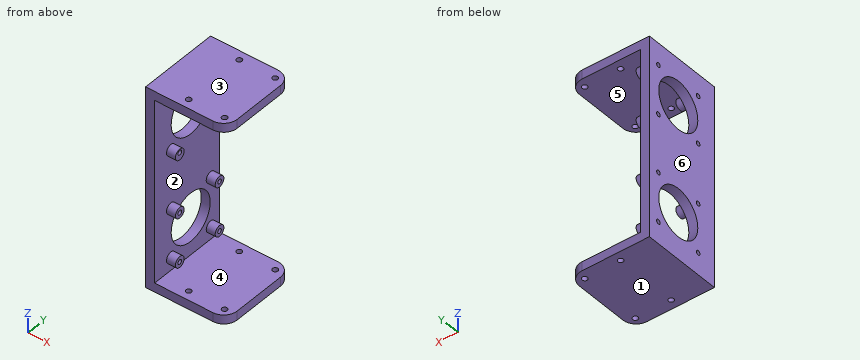
Autodesk Inventor part; units mm, degrees
ref_plane "Work Plane2" through (0, 0, 56) normal (0, 0, -1) x (-1, 0, 0)
ref_plane "YZ Plane" through (0, 0, 0) normal (1, 0, 0) x (0, 1, 0)
ref_plane "XZ Plane" through (0, 0, 0) normal (0, 1, 0) x (-1, 0, 0)
sketch "Sketch1" plane through (0, 0, 0) normal (0, 0, 1) x (1, 0, 0)
  line L0 (0, 0) -> (20, 0)
  line L1 (20, 0) -> (20, 35)
  line L2 (20, 35) -> (0, 35)
  line L3 (0, 35) -> (0, 0)
  circle A0 centre (0, 35) radius 1.5
  circle A1 centre (20, 35) radius 1.5
  circle A2 centre (0, 0) radius 1.5
  circle A3 centre (20, 0) radius 1.5
  line L4 (0, 35) -> (20, 0)
  line L5 (-15, -5) -> (20, -5)
  line L6 (20, -5) -> (20, 40)
  line L7 (20, 40) -> (-15, 40)
  line L8 (-15, 40) -> (-15, -5)
  line L9 (20, 40) -> (25, 40)
  line L10 (25, 40) -> (25, -5)
  line L11 (25, -5) -> (20, -5)
  line L12 (20, -5) -> (20, 40)
  point P0 (10, 17.5)
  point P1 (20, 36.5)
  point P2 (20, 33.5)
  point P3 (20, 1.5)
  point P4 (20, -1.5)
  dimension "d0" = 35
  dimension "d1" = 20
  dimension "d2" = 3
  dimension "d3" = 3
  dimension "d4" = 3
  dimension "d5" = 3
  dimension "d6" = 5
  dimension "d7" = 15
  dimension "d45" = 5
  dimension "d46" = 45
  dimension "d47" = 10
extrude "Extrusion1" add sketch "Sketch1" along normal blind 5 contours A2 L3 A0 L4 A3 L0 | L0 A3 L6 L5 L8 L7 A1 L2 A0 L3 A2 | L4 A0 L2 A1 L1 A3 | A3 L1 A1 L6 L9 L10 L11
sketch "Sketch2" plane through (0, 0, 5) normal (0, 0, 1) x (1, 0, 0)
  line L0 (30, 40) -> (-15, 40)
  line L1 (-15, 40) -> (-20, 40)
  line L2 (-20, 40) -> (-20, -5)
  line L3 (-20, -5) -> (-15, -5)
  line L4 (-15, -5) -> (-15, 40)
  point P0 (0, 0)
  dimension "d10" = 5
extrude "Extrusion2" add sketch "Sketch2" along normal blind 107 and the other way blind 5
ref_plane "Work Plane2" through (0, 0, 56) normal (0, 0, -1) x (-1, 0, 0)
mirror "Mirror2" about plane through (0, 0, 56) normal (0, 0, -1) of "Extrusion1"
sketch "Sketch3" plane through (-15, -5, 5) normal (1, 0, 0) x (0, 0, -1)
  line L0 (-102, 45) -> (-102, 0)
  line L1 (-102, 25) -> (0, 25)
  line L2 (0, 45) -> (0, 0)
  circle A0 centre (-81, 25) radius 13.5
  circle A1 centre (-21, 25) radius 13.5
  line L3 (-94.75, 38.75) -> (-67.25, 38.75)
  line L4 (-67.25, 38.75) -> (-67.25, 11.25)
  line L5 (-67.25, 11.25) -> (-94.75, 11.25)
  line L6 (-94.75, 11.25) -> (-94.75, 38.75)
  line L7 (-94.75, 38.75) -> (-67.25, 11.25) construction
  line L8 (-67.25, 38.75) -> (-94.75, 11.25) construction
  line L9 (0, 45) -> (-102, 45)
  line L10 (-7.25, 11.25) -> (-34.75, 11.25)
  line L11 (-34.75, 11.25) -> (-34.75, 38.75)
  line L12 (-34.75, 38.75) -> (-7.25, 38.75)
  line L13 (-7.25, 38.75) -> (-7.25, 11.25)
  line L14 (-7.25, 11.25) -> (-34.75, 38.75) construction
  line L15 (-34.75, 11.25) -> (-7.25, 38.75) construction
  circle A2 centre (-94.75, 38.75) radius 3
  circle A3 centre (-67.25, 38.75) radius 3
  circle A4 centre (-67.25, 11.25) radius 3
  circle A5 centre (-94.75, 11.25) radius 3
  circle A6 centre (-34.75, 38.75) radius 3
  circle A7 centre (-7.25, 38.75) radius 3
  circle A8 centre (-7.25, 11.25) radius 3
  circle A9 centre (-34.75, 11.25) radius 3
  circle A10 centre (-94.75, 38.75) radius 1.25
  circle A11 centre (-67.25, 38.75) radius 1.25
  circle A12 centre (-68.25, 11.25) radius 1.25
  circle A13 centre (-94.75, 11.25) radius 1.25
  circle A14 centre (-34.75, 38.75) radius 1.25
  circle A15 centre (-7.25, 38.75) radius 1.25
  circle A16 centre (-34.75, 11.25) radius 1.25
  circle A17 centre (-7.25, 11.25) radius 1.25
  point P0 (5, 5)
  dimension "d16" = 27
  dimension "d17" = 27
  dimension "d18" = 27.5
  dimension "d19" = 27.5
  dimension "d20" = 20
  dimension "d21" = 21
  dimension "d22" = 21
  dimension "d23" = 27.5
  dimension "d24" = 27.5
  dimension "d25" = 6
  dimension "d26" = 6
  dimension "d27" = 6
  dimension "d28" = 6
  dimension "d29" = 6
  dimension "d30" = 6
  dimension "d31" = 6
  dimension "d32" = 6
  dimension "d33" = 2.5
  dimension "d34" = 2.5
  dimension "d35" = 2.5
  dimension "d36" = 2.5
  dimension "d37" = 2.5
  dimension "d38" = 2.5
  dimension "d39" = 2.5
  dimension "d40" = 2.5
extrude "Extrusion3" cut sketch "Sketch3" against normal blind 6 contours A0 L1 | L1 A0 | A13 L5 L6 | L6 L5 A13 | A10 L3 L6 | L6 L3 A10 | A1 L1 | L1 A1 | A15 L12 L13 | L13 L12 A15 | A17 L10 L13 | L13 L10 A17 | A12 L4 L5 | L5 L4 A12 | A11 L4 L3 | L3 L4 A11 | A14 L11 L12 | L12 L11 A14 | A16 L11 L10 | L10 L11 A16
extrude "Extrusion4" add sketch "Sketch3" along normal blind 5 contours A5 L5 A13 L6 | L6 A13 L5 A5 | A2 L3 A10 L6 | L6 A10 L3 A2 | A7 L12 A15 L13 | L13 A15 L12 A7 | A8 L10 A17 L13 | L13 A17 L10 A8 | A4 L4 A12 L5 | L5 A12 L4 A4 | A3 L4 A11 L3 | L3 A11 L4 A3 | A6 L11 A14 L12 | L12 A14 L11 A6 | A9 L11 A16 L10 | L10 A16 L11 A9
fillet "Fillet2" radius 7.5 4 edges at (25, 40, 2.5) (25, -5, 2.5) (25, -5, 109.5) (25, 40, 109.5)
equation "\"d41\" = d30"
properties part number "StereoVisionHolder_3"
Verification items for the finished model (mm, model axes). Face numbers are marked on the shaded views. A direction names the side the tool comes from. Give positions to 0.01 mm unless a question says otherwise; leave off trailing zeros. Order: outer loops, then holes, each group sorted by start corner. A loop starts at its lowest first (then second) coordinate and runs counter-clockwise, first axis right, second up. Notation, with made-up numbers: (15, 13.5) - (58, 13.5) arc R15 cw to (58, 38.5) - close; hole circle Ø11 at (48, -30.75). An arc over 180 degrees is marked (long way). Answer as CSV lines item,"result". Start each with the question number.
Item 1: Gauge pin test, flat ends, axial feed: pin 1 (8 mm diameter, centred on x = -2.5, y = 11, fed in from -Z); pin 2 (2.5 mm diameter, centred on x = 20, y = 0, fed in from -Z); pin 3 (1.8 mm diameter, centred on y = 5, z = 39.5, fed in from +X); pin 4 (1.5 mm diameter, centred on y = 23, z = 57, fed in from +X). Record the tip position at first contact, or that the pin passes through.
Item 2: Section check C-C, the plane z = 26. Record the boundary of the cut face in (x, y), plus the area to 3 significant figures.
Item 3: Section check D-D, the plane y = 0. Record the boundary of the cut face in (x, z).
Item 4: Section check A-A, the plane x = 16. Record the boundary of the cut face in (y, z), plus the area to 3 significant figures.
Item 5: Access from +Z, -Z, +X, -X, +Y, -Y to the whole of each face (thin tool, end or side, straight path). Record for the marked faces 5 and 6.
Item 6: Mould release check, pull along Z, two halves, no side actions. Record for the marked faces 1, 2, 3 and 4: released by +Z, released by -Z, zero draft, split by the parting line, or undercut.
Item 7: Section check B-B, the plane y = 20. Record the boundary of the cut face in (x, z), plus the area to 3 significant figures.
Item 8: Material ranges on L1, parallel to Y at x = -17.25, z = 12.25; L2, parallel to Z at x = -16, y = 33.75; L3, parallel to Y at x = 0, z = 2, recorded low to high.
Filled in:
1,pin 1,"z = 0"
1,pin 2,"through"
1,pin 3,"x = -10"
1,pin 4,"x = -15"
2,outline,"(-20, -5) - (-15, -5) - (-15, 6.5) - (-20, 6.5) - close; (-20, 33.5) - (-15, 33.5) - (-15, 40) - (-20, 40) - close"
2,area,"90.0 mm^2"
3,outline,"(-20, 0) - (-1.5, 0) - (-1.5, 5) - (-15, 5) - (-15, 107) - (-1.5, 107) - (-1.5, 112) - (-20, 112) - close; (1.5, 0) - (18.5, 0) - (18.5, 5) - (1.5, 5) - close; (1.5, 107) - (18.5, 107) - (18.5, 112) - (1.5, 112) - close; (21.5, 0) - (24.57, 0) - (24.57, 5) - (21.5, 5) - close; (21.5, 107) - (24.57, 107) - (24.57, 112) - (21.5, 112) - close"
4,outline,"(-5, 0) - (40, 0) - (40, 5) - (-5, 5) - close; (-5, 107) - (40, 107) - (40, 112) - (-5, 112) - close"
4,area,"450 mm^2"
5,face 5,"+X, +Y, -Y"
5,face 6,"+Z, -Z, -X, +Y, -Y"
6,face 1,"released by -Z"
6,face 2,"undercut"
6,face 3,"released by +Z"
6,face 4,"undercut"
7,outline,"(-20, 0) - (25, 0) - (25, 5) - (-15, 5) - (-15, 12.5) - (-20, 12.5) - close; (-20, 39.5) - (-15, 39.5) - (-15, 72.5) - (-20, 72.5) - close; (-20, 99.5) - (-15, 99.5) - (-15, 107) - (25, 107) - (25, 112) - (-20, 112) - close"
7,area,"690 mm^2"
8,L1,"-5 to 5, 7.5 to 32.5, 35 to 40"
8,L2,"0 to 11, 13.5 to 38.5, 41 to 71, 73.5 to 98.5, 101 to 112"
8,L3,"-5 to -1.5, 1.5 to 33.5, 36.5 to 40"
